Design review of the part built by this model. Coordinates are the model's own, in mm. A direction names the side the tool comes from. Give positions to 0.01 mm unless a question says otherwise; leave off trailing zeros. Loops run counter-clockwise (first coordinate to the right, second up) from the corner with the lowest first, then second, coordinate; pieces in that order, holes last. Notation, with made-up numbers: (10, 68) -> (24, 68) arc R17 cw to (24, 99) -> close; hole circle Ø1 at (-23, 56). An arc over 180 degrees is marked (long way). Answer as CSV lines item,"result".
from build123d import *

# Parameters (mm, degrees)
BOSS_EXTRUDE1_DEPTH = 14.5
SKETCH1_3_R         = 1.9999999999999996
BOSS_EXTRUDE2_DEPTH = 2
SKETCH2_R           = 1.9999999999999996
BOSS_EXTRUDE3_DEPTH = 12.5
BOSS_EXTRUDE4_START = -2
SKETCH2_2_R         = 1.9999999999999996
BOSS_EXTRUDE4_DEPTH = 2
BOSS_EXTRUDE5_DEPTH = 5
CHAMFER1_SIZE       = 1.5
FILLET3_R           = 2
FILLET1_R           = 0.6
FILLET4_R           = 2
FILLET5_R           = 0.2
FILLET6_R           = 1
FILLET7_R           = 10


with BuildPart() as part:
    # Sketch1 → Boss-Extrude1 (new body)
    with BuildSketch(Plane(origin=(0, 0, 0), x_dir=(1, 0, 0), z_dir=(0, 1, 0))):
        with BuildLine():
            ThreePointArc((33, 12), (33.8, 6), (33, 0))
            Line((33, 0), (16.499999999999837, -2.00000000000002))
            Line((16.499999999999837, -2.00000000000002), (0, 0))
            ThreePointArc((0, 0), (-0.7999999999999936, 5.999999999999997), (0, 12))
            Line((0, 12), (16.499999999999837, 13.99999999999998))
            Line((16.499999999999837, 13.99999999999998), (33, 12))
        make_face()
        with BuildLine():
            Line((16.49999999999997, 12.589752836725182), (31.673748690170243, 10.750510571250008))
            ThreePointArc((31.673748690170243, 10.750510571250008), (32.39999999999999, 5.999999999999953), (31.673748690170243, 1.2494894287498812))
            Line((31.673748690170243, 1.2494894287498812), (16.49999999999984, -0.5897528367253209))
            Line((16.49999999999984, -0.5897528367253209), (1.3262513098297308, 1.2494894287498826))
            ThreePointArc((1.3262513098297308, 1.2494894287498826), (0.5999999999999286, 5.999999999999944), (1.3262513098297308, 10.750510571250004))
            Line((1.3262513098297308, 10.750510571250004), (16.49999999999997, 12.589752836725182))
        make_face(mode=Mode.SUBTRACT)
    extrude(amount=BOSS_EXTRUDE1_DEPTH)

    # Sketch1<3> → Boss-Extrude2 (add)
    with BuildSketch(Plane(origin=(0, 0, 0), x_dir=(1, 0, 0), z_dir=(0, 1, 0))):
        with BuildLine():
            ThreePointArc((31.673748690170243, 10.750510571250008), (32.39999999999999, 5.999999999999953), (31.673748690170243, 1.2494894287498812))
            Line((31.673748690170243, 1.2494894287498812), (16.49999999999984, -0.5897528367253209))
            Line((16.49999999999984, -0.5897528367253209), (1.3262513098297308, 1.2494894287498826))
            ThreePointArc((1.3262513098297308, 1.2494894287498826), (0.5999999999999286, 5.999999999999944), (1.3262513098297308, 10.750510571250004))
            Line((1.3262513098297308, 10.750510571250004), (16.49999999999997, 12.589752836725182))
            Line((16.49999999999997, 12.589752836725182), (31.673748690170243, 10.750510571250008))
        make_face()
        with Locations(Location((16.499999999999837, 5.999999999999998, 0), (0, 0, 270))):
            Circle(SKETCH1_3_R, mode=Mode.SUBTRACT)
    extrude(amount=BOSS_EXTRUDE2_DEPTH)

    # Sketch2 → Boss-Extrude3 (add)
    with BuildSketch(Plane(origin=(0, 2, 0), x_dir=(1, 0, 0), z_dir=(0, 1, 0))):
        with BuildLine():
            Line((22.34588668015035, 7.351150962268389), (25.64588668015035, 7.351150962268389))
            Line((25.64588668015035, 7.351150962268389), (25.64588668015035, 10.27237722905159))
            Line((25.64588668015035, 10.27237722905159), (17.999999999999844, 13.818181818181802))
            ThreePointArc((17.999999999999844, 13.818181818181802), (16.499999999999844, 13.999999999999986), (14.999999999999844, 13.8181818181818))
            Line((14.999999999999844, 13.8181818181818), (10.599999999999836, 11.874601321573653))
            ThreePointArc((10.599999999999836, 11.874601321573653), (9.899999999999839, 5.999999999999933), (10.599999999999838, 0.12539867842620983))
            Line((10.599999999999838, 0.12539867842620983), (14.499999999999885, -1.7575757575757784))
            Line((14.499999999999885, -1.7575757575757784), (18.499999999999837, -1.7575757575757784))
            Line((18.499999999999837, -1.7575757575757784), (18.499999999999837, 0.34314575050761753))
            ThreePointArc((18.499999999999837, 0.34314575050761753), (21.75999227294638, 3.1133962363111447), (22.34588668015035, 7.351150962268389))
        make_face()
        with Locations(Location((16.499999999999837, 5.999999999999998, 0), (0, 0, 270))):
            Circle(SKETCH2_R, mode=Mode.SUBTRACT)
    extrude(amount=BOSS_EXTRUDE3_DEPTH)

    # Sketch2<2> → Boss-Extrude4 (add)
    with BuildSketch(Plane(origin=(0, 2, 0), x_dir=(1, 0, 0), z_dir=(0, 1, 0)).offset(BOSS_EXTRUDE4_START)):
        with BuildLine():
            Line((22.34588668015035, 7.351150962268389), (25.64588668015035, 7.351150962268389))
            Line((25.64588668015035, 7.351150962268389), (25.64588668015035, 10.27237722905159))
            Line((25.64588668015035, 10.27237722905159), (17.999999999999844, 13.818181818181802))
            ThreePointArc((17.999999999999844, 13.818181818181802), (16.499999999999844, 13.999999999999986), (14.999999999999844, 13.8181818181818))
            Line((14.999999999999844, 13.8181818181818), (10.599999999999836, 11.874601321573653))
            ThreePointArc((10.599999999999836, 11.874601321573653), (9.899999999999839, 5.999999999999933), (10.599999999999838, 0.12539867842620983))
            Line((10.599999999999838, 0.12539867842620983), (14.499999999999885, -1.7575757575757784))
            Line((14.499999999999885, -1.7575757575757784), (18.499999999999837, -1.7575757575757784))
            Line((18.499999999999837, -1.7575757575757784), (18.499999999999837, 0.34314575050761753))
            ThreePointArc((18.499999999999837, 0.34314575050761753), (21.75999227294638, 3.1133962363111447), (22.34588668015035, 7.351150962268389))
        make_face()
        with Locations(Location((16.499999999999837, 5.999999999999998, 0), (0, 0, 270))):
            Circle(SKETCH2_2_R, mode=Mode.SUBTRACT)
    extrude(amount=BOSS_EXTRUDE4_DEPTH)

    # Sketch3 → Boss-Extrude5 (add)
    with BuildSketch(Plane(origin=(0, 14.5, 0), x_dir=(1, 0, 0), z_dir=(0, 1, 0))):
        with BuildLine():
            Line((22.34588668015035, 7.351150962268389), (25.64588668015035, 7.351150962268389))
            Line((25.64588668015035, 7.351150962268389), (25.64588668015035, 10.27237722905159))
            Line((25.64588668015035, 10.27237722905159), (17.999999999999826, 13.81818181818181))
            ThreePointArc((17.999999999999826, 13.81818181818181), (16.499999999999833, 13.99999999999999), (14.999999999999844, 13.818181818181802))
            Line((14.999999999999844, 13.818181818181802), (10.599999999999836, 11.874601321573653))
            ThreePointArc((10.599999999999836, 11.874601321573653), (9.899999999999842, 5.999999999999933), (10.599999999999842, 0.12539867842621155))
            Line((10.599999999999842, 0.12539867842621155), (11.173814866283609, -1.5968518966374832))
            ThreePointArc((11.173814866283609, -1.5968518966374832), (11.760910789091948, -2.4756088583346414), (12.713890329463082, -2.932473626010398))
            Line((12.713890329463082, -2.932473626010398), (14.49999999999984, -3.2568542494923824))
            Line((14.49999999999984, -3.2568542494923824), (14.49999999999984, 0.3431457505076174))
            ThreePointArc((14.49999999999984, 0.3431457505076174), (20.496967019022676, 1.5251531144804868), (22.34588668015035, 7.351150962268389))
        make_face()
        with BuildLine():
            Line((13.499999999999838, 8.599999999999934), (19.499999999999837, 8.599999999999934))
            ThreePointArc((19.499999999999837, 8.599999999999934), (20.249999999999837, 5.999999999999933), (19.499999999999837, 3.3999999999999324))
            Line((19.499999999999837, 3.3999999999999324), (13.499999999999838, 3.3999999999999324))
            ThreePointArc((13.499999999999838, 3.3999999999999324), (12.749999999999837, 5.999999999999932), (13.499999999999838, 8.599999999999934))
        make_face(mode=Mode.SUBTRACT)
    extrude(amount=BOSS_EXTRUDE5_DEPTH)

    # Chamfer1
    chamfer1_edges = [part.edges().sort_by_distance(p)[0] for p in [
        (14.49999999999984, 14.5, 0.7072150035340781),
    ]]
    chamfer(chamfer1_edges, length=CHAMFER1_SIZE)

    # Fillet3
    fillet3_edges = [part.edges().sort_by_distance(p)[0] for p in [
        (25.64588668015035, 10.75, -10.27237722905159),
    ]]
    fillet(fillet3_edges, radius=FILLET3_R)

    # Fillet1
    # the kernel refuses this fillet: 0.6 mm, written as the material it adds along each edge
    with BuildSketch(Plane(origin=(22.11701590469639, 2, -11.90890242403471), x_dir=(0.8942491782496095, 0, 0.44756944399712767), z_dir=(0, 1, 0))) as fillet1_piece_1:
        with BuildLine():
            CenterArc((3.393748585617257, 0.5763680275818249), FILLET1_R, 109.67662149320171, 144.1891632768265)
            Line((3.1917219374131016, 1.1413328348179872), (3.16141794018248, 1.2260775559034116))
            Line((3.16141794018248, 1.2260775559034116), (-0.03030399723062558, 0.08474472108542427))
            Line((-0.03030399723062558, 0.08474472108542427), (0.00268281172049191, -0.08996000512045559))
            ThreePointArc((0.00268281172049191, -0.08996000512045559), (2.614303647054314, -0.01207553882752912), (3.2020056235731444, -0.08645520413727262))
            Line((3.2020056235731444, -0.08645520413727262), (3.227015575144115, 1e-16))
        make_face()
    extrude(amount=12.5)

    # Fillet4
    # the kernel refuses this fillet: 2 mm, written as the material it adds along each edge
    with BuildSketch(Plane(origin=(18.499999999999837, 14.5, 0.34732859430107876), x_dir=(0.9927337820337083, 0, -0.12033136751923736), z_dir=(0, -1, 0))) as fillet4_piece_1:
        with BuildLine():
            CenterArc((1.5903936692052363, -2.0000000000000004), FILLET4_R, 89.99999999999994, 48.90789553913825)
            Line((0.08308572214778008, -0.6854572077191857), (0, 0))
            Line((0, 0), (1.5903936692052383, -1e-17))
        make_face()
    extrude(amount=12.5)

    # Fillet5
    fillet5_edges = [part.edges().sort_by_distance(p)[0] for p in [
        (18.499999999999837, 8.25, -0.34314575050761803),
    ]]
    fillet(fillet5_edges, radius=FILLET5_R)

    # Fillet6
    fillet6_edges = [part.edges().sort_by_distance(p)[0] for p in [
        (10.599999999999834, 17, -11.874601321573653),
    ]]
    fillet(fillet6_edges, radius=FILLET6_R)

    # Fillet7
    fillet7_edges = [part.edges().sort_by_distance(p)[0] for p in [
        (16.499999999999837, 7.25, 2.00000000000002),
    ]]
    fillet(fillet7_edges, radius=FILLET7_R)


solid = part.part
Q1. We need section C-C, the plane z = -1.75. State the section outline as (x, y) points, and give its area (3 significant figures).
Filled sheet:
outline,"(-0.4, 0) -> (33.4, 0) -> (33.4, 14.5) -> (31.82, 14.5) -> (31.82, 2) -> (20.74, 2) -> (20.74, 19.5) -> (10.26, 19.5) -> (10.26, 2) -> (1.18, 2) -> (1.18, 14.5) -> (-0.4, 14.5) -> close"
area,"290 mm^2"
Q2. We need section B-B, the plane x = 16.5. State the section outline as (y, z) points.
Filled sheet:
outline,"(0, -14) -> (19.5, -14) -> (19.5, -8.6) -> (14.5, -8.6) -> (14.5, -8) -> (0, -8) -> close; (0, -4) -> (14.5, -4) -> (14.5, -3.4) -> (19.5, -3.4) -> (19.5, 0) -> (14.5, 0) -> (14.5, 1.93) -> (0, 1.93) -> close"
Q3. For faces 1 (the cylindrical face through (14.548, 7.148, -6.434)), 2 (the flat face through (13.06, 16.96, -12.96)), 3 (the flat face through (6, 2, -6)), list the 3-axis set-ups (+Z, -Z, +X, -X, +Y, -Y) from which the entire face can be reached by the end or side of a thin tool; tool diameter is ignored.
Filled sheet:
face 1,"+Y, -Y"
face 2,"-Z, -X, +Y"
face 3,"+Y"
Q4. To check wall thickness, follow probe 1 along Z at (x, y) = (16.5, 9.5); probe 2 along X at (y, z) = (7.5, -8.75); probe 3 along X at (y, z) = (13.5, -9). State the ranges of each line that lie inside material, in increasing order. Write a range as from..to.
Filled sheet:
probe 1,"z = -14..-8, -4..1.93"
probe 2,"x = -0.63..0.84, 10.05..25.65, 32.16..33.63"
probe 3,"x = -0.6..0.89, 10.08..25.65, 32.11..33.6"
Q5. We need section A-A, the plane z = -6. State the section outline as (x, y) points.
Filled sheet:
outline,"(-0.8, 0) -> (14.5, 0) -> (14.5, 14.5) -> (12.75, 14.5) -> (12.75, 19.5) -> (9.9, 19.5) -> (9.9, 2) -> (0.6, 2) -> (0.6, 14.5) -> (-0.8, 14.5) -> close; (18.5, 0) -> (33.8, 0) -> (33.8, 14.5) -> (32.4, 14.5) -> (32.4, 2) -> (22.5, 2) -> (22.5, 19.5) -> (20.25, 19.5) -> (20.25, 14.5) -> (18.5, 14.5) -> close"
Q6. We need section D-D, the plane x = 23.5. State the section outline as (y, z) points.
Filled sheet:
outline,"(0, -13.15) -> (14.5, -13.15) -> (14.5, -11.27) -> (19.5, -11.27) -> (19.5, -7.35) -> (2, -7.35) -> (2, -0.26) -> (14.5, -0.26) -> (14.5, 1.15) -> (0, 1.15) -> close"
Q7. Clearance check with flat-ended pins moving along their axes: pin 1 Ø1.5 at (x, y) = (16, 16.5) entering from +Z; pin 2 Ø1.8 at (y, z) = (16, 1.5) entering from +X; pin 3 Ø4 at (x, y) = (27, 7) entering from +Z. State where each tip first meets the part, or that it passes through.
Filled sheet:
pin 1,"stops at z = 0"
pin 2,"stops at x = 15.4"
pin 3,"stops at z = 0.97"
Q8. The part is to be moulded in two halves that separate along X. For faces 4 (the cylindrical face through (11.75, 16.965, 2.466)), 5 (the flat face through (0.6, 14.5, -8.5)), 6 (the flat face through (16.4, 14.5, -8.3)), say which applies: pulls with the +X half, pulls with the -X half, needs draft (parallel to the pull), parting line crosses it, or undercut.
Filled sheet:
face 4,"pulls with the -X half"
face 5,"needs draft"
face 6,"undercut"
